Model file for the job. Use its own axes, mm. A direction names the side the tool comes from. Round coordinates to 2 decimals unless told otherwise and drop trailing zeros. Order: outer loops, then holes, each group sorted by start corner. A loop starts at its lowest first (then second) coordinate and runs counter-clockwise, first axis right, second up. Notation, with made-up numbers: (37.25, 64.25) - (76.25, 64.25) arc R8 cw to (76.25, 78.25) - close; hole circle Ø10 at (31, -2). An arc over 180 degrees is marked (long way). Use one line per item in the form item = value.
from build123d import *

# Parameters (mm, degrees)
F0_R     = 12.5
F1_DEPTH = 10
F2_R     = 6
F3_DEPTH = 7.5


with BuildPart() as f1:
    # F0 (on Top) → F1 (new body, symmetric)
    with BuildSketch(Plane.XY):
        with BuildLine():
            Line((24.387505, 12.5), (-24.387505, 12.5))
            ThreePointArc((-24.387505, 12.5), (-60, 0), (-24.387505, -12.5))
            Line((-24.387505, -12.5), (24.387505, -12.5))
            ThreePointArc((24.387505, -12.5), (60, 0), (24.387505, 12.5))
        make_face()
        with Locations((-40, 0)):
            Circle(F0_R, mode=Mode.SUBTRACT)
        with Locations((40, 0)):
            Circle(F0_R, mode=Mode.SUBTRACT)
    extrude(amount=F1_DEPTH, both=True)

    # F2 (on Right) → F3 (join, symmetric)
    with BuildSketch(Plane.YZ):
        with BuildLine():
            Line((12.5, -10), (-12.5, -10))
            Line((-12.5, -10), (-12.5, -30))
            ThreePointArc((-12.5, -30), (0, -42.5), (12.5, -30))
            Line((12.5, -30), (12.5, -10))
        make_face()
        with Locations((0, -30)):
            Circle(F2_R, mode=Mode.SUBTRACT)
    extrude(amount=F3_DEPTH, both=True)


solid = f1.part
(1) Tool access for faces 1 (the face through (0.105, -0.275, -42.497)), 2 (the face through (0, -12.5, -5)), 3 (the face through (0, 12.5, -5)), 4 (the face through (28, 5, -10)), 5 (the face through (-28, 5, -10)): list every direction of +Z, -Z, +X, -X, +Y, -Y with a clear straight run to the whole face (end or side of a thin tool).
Report:
face_1 = -Z, +X, -X
face_2 = +Z, -Z, -Y
face_3 = +Z, -Z, +Y
face_4 = -Z, +X, +Y, -Y
face_5 = -Z, -X, +Y, -Y
(2) Slice it at C-C on z = 4. Give the cut face in (x, y), then the cut area to 3 significant figures.
Report:
outline = (-24.39, -12.5) - (24.39, -12.5) arc R20 ccw (long way) to (24.39, 12.5) - (-24.39, 12.5) arc R20 ccw (long way) to start; hole circle Ø25 at (-40, 0); hole circle Ø25 at (40, 0)
area = 2,600 mm2
(3) Slice it at B-B on x = 40. Give the cut face in (y, z), then the cut area to 3 significant figures.
Report:
outline = (-20, -10) - (-12.5, -10) - (-12.5, 10) - (-20, 10) - close; (12.5, -10) - (20, -10) - (20, 10) - (12.5, 10) - close
area = 300 mm2
(4) Pin check, flat tips, straight feed: pin 1 (10 mm diameter, centred on y = -8, z = -5.5, fed in from +X); pin 2 (20 mm diameter, centred on y = -5, z = -26.5, fed in from +X); pin 3 (10 mm diameter, centred on x = 47.5, y = 1.5, fed in from -Z); pin 4 (10 mm diameter, centred on x = 45, y = -10, fed in from +Z). Stop position of each tip, or through.
Report:
pin_1 = 59.77
pin_2 = 7.5
pin_3 = -10
pin_4 = 10
(5) Probe probe 1 along X at (y, z) = (-0.5, -9.5); probe 2 along Y at (x, z) = (-40, 2.25); probe 3 along Z at (x, y) = (-1, 0). List the from-to ranges inside material, lowest first. Write a range as [from, to].
Report:
probe_1 = [-59.99, -52.49], [-27.51, 27.51], [52.49, 59.99]
probe_2 = [-20, -12.5], [12.5, 20]
probe_3 = [-42.5, -36], [-24, 10]
(6) Slice it at D-D on y = -16. Give the cut face in (x, z), then the cut area to 3 significant figures.
Report:
outline = (-52, -10) - (-28, -10) - (-28, 10) - (-52, 10) - close; (28, -10) - (52, -10) - (52, 10) - (28, 10) - close
area = 960 mm2
(7) Slice it at A-A on y = 0. Give the cut face in (x, z), then the cut area to 3 significant figures.
Report:
outline = (-60, -10) - (-52.5, -10) - (-52.5, 10) - (-60, 10) - close; (-27.5, -10) - (-7.5, -10) - (-7.5, -24) - (7.5, -24) - (7.5, -10) - (27.5, -10) - (27.5, 10) - (-27.5, 10) - close; (-7.5, -42.5) - (7.5, -42.5) - (7.5, -36) - (-7.5, -36) - close; (52.5, -10) - (60, -10) - (60, 10) - (52.5, 10) - close
area = 1,710 mm2
(8) Pull direction X, two halves, no side cores. Call faces 6 (the face through (27.512, 0.55, -0.14)), 7 (the face through (-0.105, -1.301, -35.857)), 8 (the face through (-7.5, 0, -22)), 9 (the face through (-59.99, 0.69, 0.14)): released by +X, released by -X, zero draft, split by the parting line, or undercut.
Report:
face_6 = undercut
face_7 = zero draft
face_8 = released by -X
face_9 = undercut
